```python
from build123d import *

# Parameters (mm, degrees)
SKETCH1_W           = 66.548
SKETCH1_H           = 96.774
SKETCH1_R           = 19.05
SKETCH1_R_2         = 4
BOSS_EXTRUDE3_DEPTH = 3.175
SKETCH3_W           = 50.8
SKETCH3_H           = 96.774
SKETCH3_R           = 2.7432
BOSS_EXTRUDE4_DEPTH = 3.175
FILLET2_R           = 1.016
FILLET3_R           = 4.191


with BuildPart() as part:
    # Sketch1 → Boss-Extrude3 (new body)
    with BuildSketch(Plane.XY):
        with Locations((0, 15.113)):
            Rectangle(SKETCH1_W, SKETCH1_H)
        Circle(SKETCH1_R, mode=Mode.SUBTRACT)
        with Locations((23.5, 23.5)):
            Circle(SKETCH1_R_2, mode=Mode.SUBTRACT)
        with Locations((23.5, -23.5)):
            Circle(SKETCH1_R_2, mode=Mode.SUBTRACT)
        with Locations((-23.5, -23.5)):
            Circle(SKETCH1_R_2, mode=Mode.SUBTRACT)
        with Locations((-23.5, 23.5)):
            Circle(SKETCH1_R_2, mode=Mode.SUBTRACT)
    extrude(amount=BOSS_EXTRUDE3_DEPTH)

    # Sketch3 → Boss-Extrude4 (add)
    with BuildSketch(Plane.ZY.offset(33.274)):
        with Locations((25.4, 15.113)):
            Rectangle(SKETCH3_W, SKETCH3_H)
        with Locations(Location((38.1, 50.8, 0), (0, 0, 270))):
            Circle(SKETCH3_R, mode=Mode.SUBTRACT)
        with Locations(Location((12.7, 50.8, 0), (0, 0, 270))):
            Circle(SKETCH3_R, mode=Mode.SUBTRACT)
        with Locations(Location((38.1, 25.4, 0), (0, 0, 270))):
            Circle(SKETCH3_R, mode=Mode.SUBTRACT)
        with Locations(Location((12.7, 25.4, 0), (0, 0, 270))):
            Circle(SKETCH3_R, mode=Mode.SUBTRACT)
        with Locations(Location((38.1, 0, 0), (0, 0, 270))):
            Circle(SKETCH3_R, mode=Mode.SUBTRACT)
        with Locations(Location((12.7, 0, 0), (0, 0, 270))):
            Circle(SKETCH3_R, mode=Mode.SUBTRACT)
    extrude(amount=-BOSS_EXTRUDE4_DEPTH)

    # Fillet2
    fillet2_edges = [part.edges().sort_by_distance(p)[0] for p in [
        (-30.099, 15.113, 3.175),
    ]]
    fillet(fillet2_edges, radius=FILLET2_R)

    # Fillet3
    fillet3_edges = [part.edges().sort_by_distance(p)[0] for p in [
        (-33.274, 15.113, 0),
    ]]
    fillet(fillet3_edges, radius=FILLET3_R)


solid = part.part
```
CAD build for the part. Positions are in the model's coordinates, mm. A direction names the side the tool comes from. Round coordinates to 2 decimals unless told otherwise and drop trailing zeros. Order: outer loops, then holes, each group sorted by start corner. A loop starts at its lowest first (then second) coordinate and runs counter-clockwise, first axis right, second up. Notation, with made-up numbers: (56, 20.25) - (76, 20.25) arc R14 ccw to (76, 30.25) - close; hole circle Ø4 at (12, 36). An arc over 180 degrees is marked (long way). Answer in a Markdown table with one row per item. Add a question column.
(1) Band-saw the part on C-C on z = 38.1. List the corners of the cut face in (x, y), and give its area (3 significant figures).
(2) Band-saw the part on D-D on y = 0. List the corners of the cut face in (x, z) (3 decimals), and give its area (3 significant figures).
(3) Mould opens along Z. For faces 3 (the face through (-10, 63.5, 3)), 4 (the face through (-31.709, -1.475, 15.013)), 5 (the face through (-31.709, 48.183, 38.924)), 6 (the face through (2, 27, 3.175)) say: +Z half, -Z half, draft (parallel to the pull), parting line (faces both ways), or undercut.
(4) Drop flat-ended pins along their axis: pin 1 Ø3 at (x, y) = (5.5, -17.5) entering from +Z (3 decimals); pin 2 Ø1.5 at (y, z) = (53.5, 7.5) entering from +X. Give the stop position or say it passes through.
(5) Band-saw the part on A-A on y = -23.5. List the corners of the cut face in (x, z) (3 decimals).
(6) Band-saw the part on B-B on x = 0. List the corners of the cut face in (y, z) (3 decimals), and give its area (3 significant figures).
(7) 3-axis set-ups, long thin cutter, end or side, ignore diameter. For faces 1 (the face through (-31.709, 23.925, 40.413)), 2 (the face through (-30.099, 16, 27)): which of +Z, -Z, +X, -X, +Y, -Y reach the whole face in a straight line?
(8) Probe L1, parallel to X at y = -28.5, z = 42; L2, parallel to Z at x = -11.5, y = -21 (3 decimals); L3, parallel to Z at x = -32.2, y = 50.8. List the from-to ranges inside material, lowest first. Write a range as [from, to].
Data:
| question | item | result |
|---|---|---|
| 1 | outline | (-33.27, -33.27) - (-30.1, -33.27) - (-30.1, -2.74) - (-33.27, -2.74) - close; (-33.27, 2.74) - (-30.1, 2.74) - (-30.1, 22.66) - (-33.27, 22.66) - close; (-33.27, 28.14) - (-30.1, 28.14) - (-30.1, 48.06) - (-33.27, 48.06) - close; (-33.27, 53.54) - (-30.1, 53.54) - (-30.1, 63.5) - (-33.27, 63.5) - close |
| 1 | area | 255 mm^2 |
| 2 | outline | (-33.274, 4.191) arc R4.191 ccw to (-29.083, 0) - (-19.05, 0) - (-19.05, 3.175) - (-29.083, 3.175) arc R1.016 cw to (-30.099, 4.191) - (-30.099, 9.957) - (-33.274, 9.957) - close; (-33.274, 15.443) - (-30.099, 15.443) - (-30.099, 35.357) - (-33.274, 35.357) - close; (-33.274, 40.843) - (-30.099, 40.843) - (-30.099, 50.8) - (-33.274, 50.8) - close; (19.05, 0) - (33.274, 0) - (33.274, 3.175) - (19.05, 3.175) - close |
| 2 | area | 203 mm^2 |
| 3 | face 3 | draft |
| 3 | face 4 | undercut |
| 3 | face 5 | undercut |
| 3 | face 6 | +Z half |
| 4 | pin 1 | stops at z = 3.175 |
| 4 | pin 2 | stops at x = -30.1 |
| 5 | outline | (-33.274, 4.191) arc R4.191 ccw to (-29.083, 0) - (-27.5, 0) - (-27.5, 3.175) - (-29.083, 3.175) arc R1.016 cw to (-30.099, 4.191) - (-30.099, 50.8) - (-33.274, 50.8) - close; (-19.5, 0) - (19.5, 0) - (19.5, 3.175) - (-19.5, 3.175) - close; (27.5, 0) - (33.274, 0) - (33.274, 3.175) - (27.5, 3.175) - close |
| 6 | outline | (-33.274, 0) - (-19.05, 0) - (-19.05, 3.175) - (-33.274, 3.175) - close; (19.05, 0) - (63.5, 0) - (63.5, 3.175) - (19.05, 3.175) - close |
| 6 | area | 186 mm^2 |
| 7 | face 1 | +X, -X |
| 7 | face 2 | +Z, +X, +Y, -Y |
| 8 | L1 | x = [-33.27, -30.1] |
| 8 | L2 | z = [0, 3.175] |
| 8 | L3 | z = [1.39, 9.96], [15.44, 35.36], [40.84, 50.8] |
